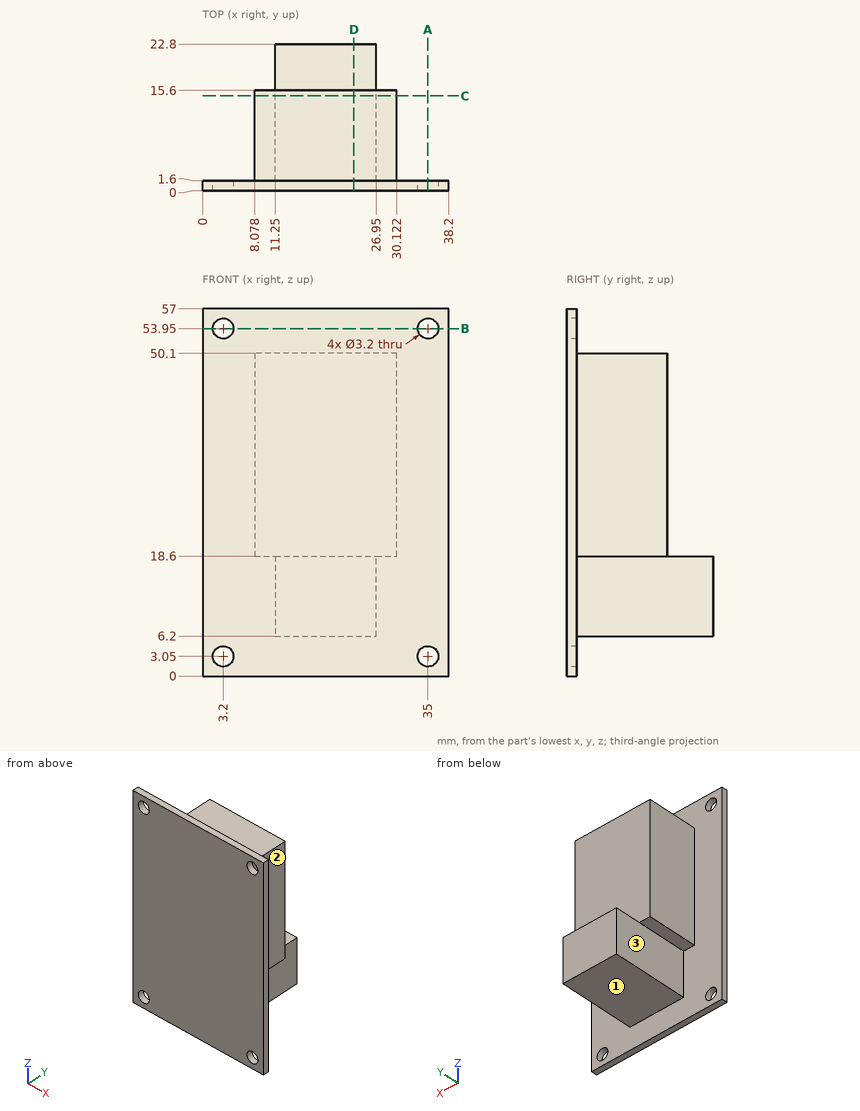
Design review of the part shown in the three views and the two pictorial views. Dimensions are in mm from the part's minimum x, y and z. A direction names the side the tool comes from. Coordinates: 2 decimals unless noted, no trailing zeros. Order: outer loops, then holes, each group sorted by start corner. A loop starts at its lowest first (then second) coordinate and runs counter-clockwise, first axis right, second up.
1) Take a section at A-A, the plane x = 35. Give the boundary of the cut face in (y, z).
2) Clearance check with flat-ended pins moving along their axes: pin 1 (2 mm diameter, centred on x = 22, y = 18.5, fed in from +Z); pin 2 (4 mm diameter, centred on x = 3.2, z = 3.05, fed in from +Y); pin 3 (3.5 mm diameter, centred on y = 15, z = 11.5, fed in from +X). State where each tip first meets the part, or that it passes through.
3) Take a section at B-B, the plane z = 53.95. Give the boundary of the cut face in (x, y).
4) Wall thickness on line 1 along Z through (x, y) = (3.2, 1.2); line 2 along Z through (x, y) = (27, 12.25); line 3 along Y through (x, z) = (18.5, 51): over which ranges is each line inside the solid? List them lowest first.
5) Take a section at D-D, the plane x = 23.5. Give the boundary of the cut face in (y, z), and give its area (3 significant figures).
6) For the marked faces 1, 2 and 3, list the 3-axis set-ups (+Z, -Z, +X, -X, +Y, -Y) from which the entire face can be reached by the end or side of a thin tool; tool diameter is ignored.
7) Take a section at C-C, the plane y = 14.75. Give the boundary of the cut face in (x, z), and give its area (3 significant figures).
Returned:
1. outline: (0, 0) - (1.6, 0) - (1.6, 1.45) - (0, 1.45) - close; (0, 4.65) - (1.6, 4.65) - (1.6, 52.35) - (0, 52.35) - close; (0, 55.55) - (1.6, 55.55) - (1.6, 57) - (0, 57) - close
2. pin 1: stops at z = 18.6
2. pin 2: stops at y = 1.6
2. pin 3: stops at x = 26.95
3. outline: (0, 0) - (1.6, 0) - (1.6, 1.6) - (0, 1.6) - close; (4.8, 0) - (33.4, 0) - (33.4, 1.6) - (4.8, 1.6) - close; (36.6, 0) - (38.2, 0) - (38.2, 1.6) - (36.6, 1.6) - close
4. line 1: z = 0 to 1.45, 4.65 to 52.35, 55.55 to 57
4. line 2: z = 18.6 to 50.1
4. line 3: y = 0 to 1.6
5. outline: (0, 0) - (1.6, 0) - (1.6, 6.2) - (22.8, 6.2) - (22.8, 18.6) - (15.6, 18.6) - (15.6, 50.1) - (1.6, 50.1) - (1.6, 57) - (0, 57) - close
5. area: 795 mm2
6. face 1: -Z, +X, -X, +Y
6. face 2: +Z, -Z, +X, +Y
6. face 3: -Z, -X, +Y
7. outline: (8.08, 18.6) - (11.25, 18.6) - (11.25, 6.2) - (26.95, 6.2) - (26.95, 18.6) - (30.12, 18.6) - (30.12, 50.1) - (8.08, 50.1) - close
7. area: 889 mm2
